```python
from build123d import *

# Parameters (mm, degrees)
SKETCH_1_W      = 10
SKETCH_1_H      = 10
SKETCH_1_W_2    = 8
SKETCH_1_H_2    = 8
EXTRUDE_1_DEPTH = 80.155
HOLE_WIZARD_1_D = 3


with BuildPart() as part:
    # 草图1 → 凸台-拉伸1 (new, symmetric)
    with BuildSketch(Plane.XY):
        Rectangle(SKETCH_1_W, SKETCH_1_H)
        Rectangle(SKETCH_1_W_2, SKETCH_1_H_2, mode=Mode.SUBTRACT)
    extrude(amount=EXTRUDE_1_DEPTH, both=True)

    # 孔1 (through all)
    with Locations(Plane(origin=(0, -5, 0), x_dir=(-1, 0, 0), z_dir=(0, -1, 0))):
        with Locations((0.003475522, -41.312740983), (0.003475522, 41.312740983)):
            Hole(HOLE_WIZARD_1_D / 2)


solid = part.part
```
The listing builds one solid part. Answer for the finished solid, in the listing's coordinates (mm). A direction names the side the tool comes from. Give positions to 0.01 mm unless a question says otherwise; leave off trailing zeros. Order: outer loops, then holes, each group sorted by start corner. A loop starts at its lowest first (then second) coordinate and runs counter-clockwise, first axis right, second up. Notation, with made-up numbers: (-25.75, 82.5) -> (6.25, 82.5) arc R25 cw to (6.25, 98.5) -> close; hole circle Ø5 at (5, 67.25). An arc over 180 degrees is marked (long way). Write each question's results on one line, items separated by ' | '.
Q1. Determine the mould class of faces 3 (the face through (-4, 0, 1)), 4 (the face through (5, 0, 1)), 5 (the face through (0, 5, 1)), 6 (the face through (-5, 0, 1)) for opening direction X: pulls with the +X half, pulls with the -X half, needs draft (parallel to the pull), parting line crosses it, or undercut.
Checked values:
face 3: undercut | face 4: pulls with the +X half | face 5: needs draft | face 6: pulls with the -X half
Q2. A straight line is drawn through the part: probe 1 along X at (y, z) = (2.75, -43). Find the intervals that lie inside material, in ascending order. Write a range as from..to.
Checked values:
probe 1: x = -5..-4, 4..5
Q3. Which of the six approach directions +Z, -Z, +X, -X, +Y, -Y give full straight-line access (tool end or side, diameter ignored) to faces 1 (the face through (-0.329, 4.507, 42.777)), 2 (the face through (0, -4, 1))?
Checked values:
face 1: +Y, -Y | face 2: +Z, -Z
Q4. The part is cut by section A-A, the plane y = -0.5. Give the vertices of the cut face in (x, z) (3 decimals), and give its area (3 significant figures).
Checked values:
outline: (-5, -80.155) -> (-4, -80.155) -> (-4, 80.155) -> (-5, 80.155) -> close; (4, -80.155) -> (5, -80.155) -> (5, 80.155) -> (4, 80.155) -> close | area: 321 mm^2
Q5. This flat-tipped pin is pushed along its axis until it touches: P1, Ø3.5, axis at x = 0, z = 41.31, coming from the +Y side. Where does it stop, or does it pass through?
Checked values:
P1: stops at y = 5
Q6. The part is cut by section B-B, the plane z = 57. Give the vertices of the cut face in (x, y), and give its area (3 significant figures).
Checked values:
outline: (-5, -5) -> (5, -5) -> (5, 5) -> (-5, 5) -> close; hole (-4, -4) -> (4, -4) -> (4, 4) -> (-4, 4) -> close | area: 36.0 mm^2
